Verification items for this drawing (mm, ordinates from the low corner). A direction names the side the tool comes from. Give positions to 0.01 mm unless a question says otherwise; leave off trailing zeros. Loops run counter-clockwise (first coordinate to the right, second up) from the corner with the lowest first, then second, coordinate; pieces in that order, holes last. Notation, with made-up numbers: (75, 84) -> (84, 84) arc R19 ccw to (84, 107) -> close; hole circle Ø9 at (23, 58.5). An arc over 180 degrees is marked (long way). Answer as CSV lines item,"result". Start each with the question number.
(1) Gauge pin test, flat ends, axial feed: pin 1 Ø2 at (x, z) = (36.5, 35.5) entering from -Y; pin 2 Ø2.5 at (x, z) = (54, 10) entering from +Y; pin 3 Ø6 at (y, z) = (49, 24.5) entering from +X. Record the tip position at first contact, or that the pin passes through.
(2) Section check C-C on z = 10. State how many separate pieces and enclosed holes the cut face has, plus the area to 3 significant figures.
(3) Release check for a two-part mould opening along Y. For the marked faces 4, 5 and 6 record: pulls with the +Y half, pulls with the -Y half, needs draft (parallel to the pull), parting line crosses it, or undercut.
(4) Material ranges on line 1 (Z direction, x = 1, y = 30); line 2 (Y direction, x = 67.5, z = 29); line 3 (X direction, y = 51, z = 3), recorded low to high. Write a range as from..to.
(5) Section check A-A on x = 54. Enter the section's corners in (y, z).
(6) Access from +Z, -Z, +X, -X, +Y, -Y to the whole of each face (thin tool, end or side, straight path). Record for the marked faces 1, 2 and 3.
(7) Section check D-D on x = 14. Enter the section's corners in (y, z), plus the area to 3 significant figures.
(8) Section check B-B on z = 25. Enter the section's corners in (x, y), plus the area to 3 significant figures.
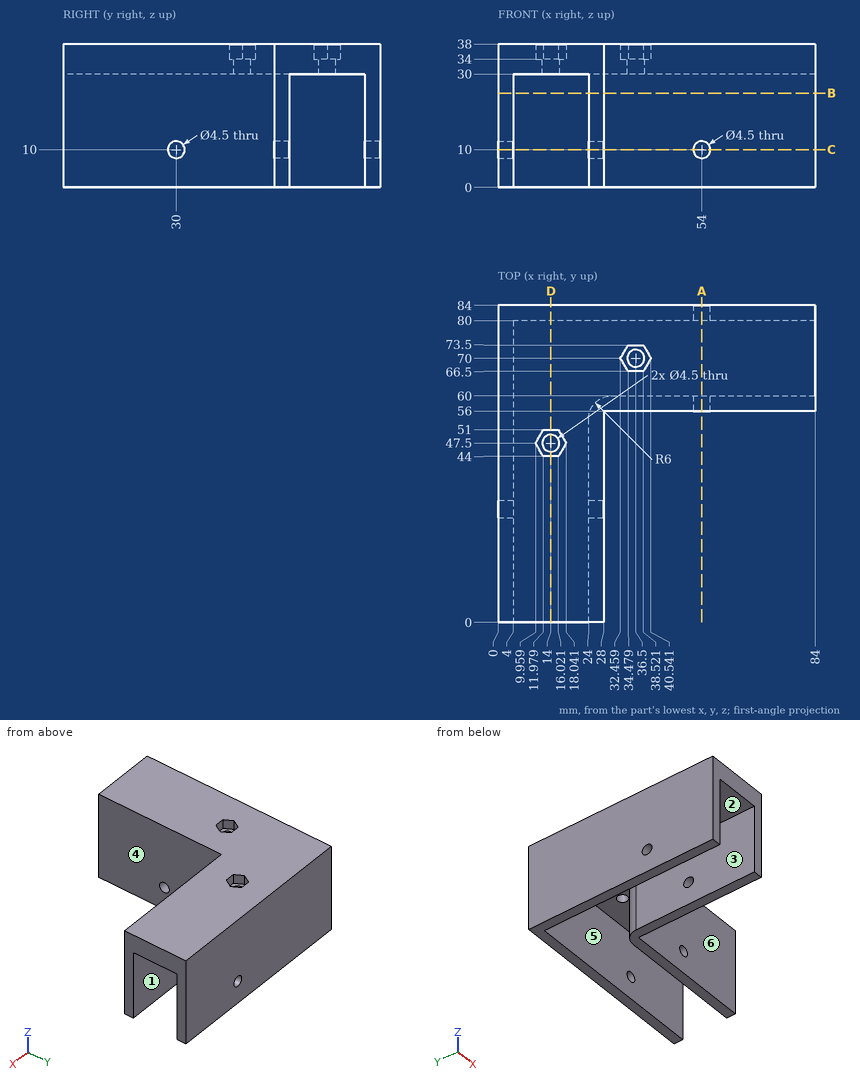
Working result:
1,pin 1,"stops at y = 56"
1,pin 2,"passes through"
1,pin 3,"stops at x = 28"
2,separate pieces,"6"
2,enclosed holes,"0"
2,area,"1,040 mm^2"
3,face 4,"needs draft"
3,face 5,"undercut"
3,face 6,"pulls with the -Y half"
4,line 1,"z = 0..7.75, 12.25..38"
4,line 2,"y = 56..60, 80..84"
4,line 3,"x = 0..4, 24..28"
5,outline,"(56, 0) -> (60, 0) -> (60, 7.75) -> (56, 7.75) -> close; (56, 12.25) -> (60, 12.25) -> (60, 30) -> (80, 30) -> (80, 12.25) -> (84, 12.25) -> (84, 38) -> (56, 38) -> close; (80, 0) -> (84, 0) -> (84, 7.75) -> (80, 7.75) -> close"
6,face 1,"-Z, +X"
6,face 2,"-Z"
6,face 3,"-Z, -Y"
7,outline,"(0, 30) -> (45.25, 30) -> (45.25, 34) -> (44, 34) -> (44, 38) -> (0, 38) -> close; (49.75, 30) -> (80, 30) -> (80, 0) -> (84, 0) -> (84, 38) -> (51, 38) -> (51, 34) -> (49.75, 34) -> close"
7,area,"746 mm^2"
8,outline,"(0, 0) -> (4, 0) -> (4, 80) -> (84, 80) -> (84, 84) -> (0, 84) -> close; (24, 0) -> (28, 0) -> (28, 56) -> (84, 56) -> (84, 60) -> (30, 60) arc R6 ccw to (24, 54) -> close"
8,area,"1,110 mm^2"
